Read the model definition and answer for the solid it produces. Units are mm, in the model's axes. A direction names the side the tool comes from. Round coordinates to 2 decimals unless told otherwise and drop trailing zeros. Answer as CSV lines item,"result".
```python
from build123d import *

# Parameters (mm, degrees)
BOSS_EXTRUDE2_DEPTH      = 71.4
BOSS_EXTRUDE2_DEPTH_BACK = 10
SKETCH7_R                = 37.5
SKETCH7_R_2              = 35.68


with BuildPart() as part:
    # Sketch6 → Revolve1 (revolve)
    with BuildSketch(Plane.XY):
        with BuildLine():
            add(Edge.make_bspline(
                [(0, 0.000773686), (0.345837081, 0.097913039), (1.048861774, 0.294893917), (2.658804783, 0.744910728), (4.053557927, 1.130839742), (5.859110481, 1.629238964), (7.4449339, 2.063004405), (9.561107041, 2.639174776), (12.031731905, 3.305427777), (14.95864462, 4.086722796), (18.28128803, 4.961677348), (21.619538634, 5.829353926), (25.788137705, 6.898189705), (30.800356023, 8.160252936), (35.816708136, 9.394330637), (40.841342365, 10.601594193), (45.87030729, 11.786766239), (50.904823346, 12.9501928), (56.785447795, 14.275517838), (65.198696746, 16.114081378), (73.627596987, 17.879432312), (82.07158253, 19.571461259), (92.221500813, 21.513709315), (109.165721029, 24.603653307), (127.869230818, 27.637744384), (146.634286906, 30.26464954), (163.735036766, 32.318446728), (174.005722776, 33.461475939), (184.286037164, 34.515191531), (194.577348102, 35.457150565), (204.878113597, 36.287219685), (213.467762549, 36.904293409), (220.342435031, 37.353141106), (227.220133715, 37.75715841), (233.239870853, 38.071431948), (238.401716288, 38.312770004), (242.702957325, 38.49518804), (246.146416964, 38.629902708), (249.586229399, 38.753396186), (253.033645652, 38.865667159), (256.46919635, 38.966714436), (259.925366913, 39.056536942), (263.348226534, 39.135133723), (266.826889882, 39.202503943), (270.213132828, 39.258646887), (273.75770095, 39.303561958), (276.606326241, 39.333037839), (279.440738032, 39.351284936), (281.598838185, 39.363917591), (283.944232781, 39.368596368), (285.031559311, 39.370000002), (285.75, 39.370000002)],
                knots=[0.083339184, 0.083339184, 0.083339184, 0.083339184, 0.083339184, 0.088305037, 0.093270891, 0.098236744, 0.103202598, 0.108168451, 0.113134305, 0.123066011, 0.132997715, 0.142929419, 0.152861123, 0.162792827, 0.18265623, 0.202519633, 0.212451338, 0.222383043, 0.242246454, 0.262109863, 0.281973272, 0.321700076, 0.341563488, 0.3614269, 0.401153715, 0.520334158, 0.56006097, 0.579924379, 0.599787787, 0.639514601, 0.679241414, 0.699104823, 0.718968231, 0.738831638, 0.758695045, 0.778558452, 0.788490156, 0.798421859, 0.808353563, 0.818285267, 0.828216971, 0.838148675, 0.848080378, 0.858012082, 0.867943786, 0.87787549, 0.887807193, 0.897738897, 0.902704749, 0.9076706, 0.917602304, 0.917602304, 0.917602304, 0.917602304, 0.917602304], degree=4))
            Line((0, 0.000773686), (7.072205141, 0.000773686))
            add(Edge.make_bspline(
                [(7.072205141, 0.000773686), (7.37488273, 0.083491425), (8.087763714, 0.278009605), (9.668024639, 0.708007227), (12.031731905, 1.345427777), (14.95864462, 2.126722796), (18.28128803, 3.001677347), (21.619538634, 3.869353926), (25.788137705, 4.938189704), (30.800356023, 6.200252936), (35.816708136, 7.434330637), (40.841342365, 8.641594193), (45.87030729, 9.826766239), (50.904823346, 10.990192799), (56.785447795, 12.315517838), (65.198696746, 14.154081378), (73.627596987, 15.919432312), (82.07158253, 17.611461259), (92.221500813, 19.553709315), (109.165721029, 22.643653307), (127.869230818, 25.677744384), (146.634286906, 28.30464954), (163.735036766, 30.358446727), (174.005722776, 31.501475938), (184.286037164, 32.555191531), (194.577348102, 33.497150565), (204.878113597, 34.327219685), (213.467762549, 34.944293408), (220.342435031, 35.393141105), (227.220133715, 35.79715841), (233.239870853, 36.111431948), (238.401716288, 36.352770003), (242.702957325, 36.535188039), (246.146416964, 36.669902707), (249.586229399, 36.793396185), (253.033645652, 36.905667159), (256.46919635, 37.006714436), (259.925366913, 37.096536942), (263.348226534, 37.175133723), (266.826889882, 37.242503943), (270.213132829, 37.298646887), (273.75770095, 37.343561958), (276.606326242, 37.373037838), (279.440738032, 37.391284936), (281.598838185, 37.403917591), (283.944232781, 37.408596368), (285.031559311, 37.410000001), (285.75, 37.410000001)],
                knots=[0.104491997, 0.104491997, 0.104491997, 0.104491997, 0.104491997, 0.108168451, 0.113134305, 0.123066011, 0.132997715, 0.142929419, 0.152861123, 0.162792827, 0.18265623, 0.202519633, 0.212451338, 0.222383043, 0.242246454, 0.262109863, 0.281973272, 0.321700076, 0.341563488, 0.3614269, 0.401153715, 0.520334158, 0.56006097, 0.579924379, 0.599787787, 0.639514601, 0.679241414, 0.699104823, 0.718968231, 0.738831638, 0.758695045, 0.778558452, 0.788490156, 0.798421859, 0.808353563, 0.818285267, 0.828216971, 0.838148675, 0.848080378, 0.858012082, 0.867943786, 0.87787549, 0.887807193, 0.897738897, 0.902704749, 0.9076706, 0.917602304, 0.917602304, 0.917602304, 0.917602304, 0.917602304], degree=4))
            Line((285.749999997, 37.410000001), (285.749999997, 39.370000001))
        make_face()
    revolve(axis=Axis((0, 0.000773686, 0), (1, 0, 0)))

    # Sketch7 → Boss-Extrude2 (add, two sides: drawn at the far end of the back side and taken through both)
    with BuildSketch(Plane(origin=(285.749999997, 0, 0), x_dir=(0, 0, -1), z_dir=(1, 0, 0)).offset(-BOSS_EXTRUDE2_DEPTH_BACK)):
        Circle(SKETCH7_R)
        Circle(SKETCH7_R_2, mode=Mode.SUBTRACT)
    extrude(amount=BOSS_EXTRUDE2_DEPTH + BOSS_EXTRUDE2_DEPTH_BACK)


solid = part.part
```
1) A tool of negligible diameter and unlimited length cuts with its end or side. For faces 4 (the face through (315.88, -34.832, 7.735)), 5 (the face through (357.15, -14, -33)), from which of +Z, -Z, +X, -X, +Y, -Y can it reach the whole face along a straight path? Write none if from no direction.
Entries:
face 4,"+X"
face 5,"+Z, -Z, +X, +Y, -Y"
2) Find the intervals of material crossed by line 1 (Y direction, x = 325, z = 0); line 2 (Z direction, x = 274, y = 23.5); line 3 (Z direction, x = 307, y = 12.5), in increasing order.
Entries:
line 1,"y = -37.5 to -35.68, 35.68 to 37.5"
line 2,"z = -31.51 to -29.02, 29.02 to 31.51"
line 3,"z = -35.36 to -33.42, 33.42 to 35.36"
3) Each of these flat-tipped pins is pushed along its axis until it touches: P1, Ø10, axis at x = 314, y = -28.5, coming from the -Z side; P2, Ø8, axis at x = 76.5, z = 26, coming from the -Y side; P3, Ø5, axis at x = 82, y = 5.5, coming from the +Z side; P4, Ø8, axis at x = 152.5, y = 17.5, coming from the +Z side. Where does it stop, or does it pass through?
Entries:
P1,"stops at z = -29.22"
P2,"passes through"
P3,"stops at z = 19.53"
P4,"stops at z = 27.91"
4) The mould has two halves that part along Z. Classify faces 1 (the face through (320.95, 37.18, 4.88)), 2 (the face through (275.75, -33, -14)), 3 (the face through (285.75, -35, -14)): pulls with the +Z half, pulls with the -Z half, needs draft (parallel to the pull), parting line crosses it, or undercut.
Entries:
face 1,"parting line crosses it"
face 2,"undercut"
face 3,"needs draft"
